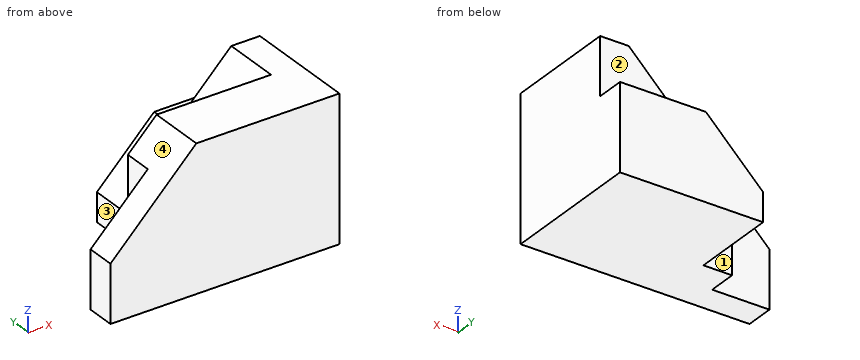
from build123d import *

# Parameters (mm, degrees)
SKETCH1_W           = 80
SKETCH1_H           = 50
BOSS_EXTRUDE1_DEPTH = 10
CUT_EXTRUDE1_DEPTH  = 10
BOSS_EXTRUDE2_DEPTH = 10
BOSS_EXTRUDE3_DEPTH = 20
BOSS_EXTRUDE4_DEPTH = 10


with BuildPart() as part:
    # Sketch1 → Boss-Extrude1 (new body)
    with BuildSketch(Plane(origin=(0, 0, 0), x_dir=(1, 0, 0), z_dir=(0, 1, 0))):
        with Locations((40, 25)):
            Rectangle(SKETCH1_W, SKETCH1_H)
    extrude(amount=BOSS_EXTRUDE1_DEPTH)

    # Sketch2 → Cut-Extrude1 (cut)
    with BuildSketch(Plane(origin=(0, 10, 0), x_dir=(1, 0, 0), z_dir=(0, 1, 0))):
        Polygon((0, 30), (30, 0), (0, 0), align=None)
    extrude(amount=-CUT_EXTRUDE1_DEPTH, mode=Mode.SUBTRACT)

    # Sketch3 → Boss-Extrude2 (add)
    with BuildSketch(Plane(origin=(0, 10, 0), x_dir=(1, 0, 0), z_dir=(0, 1, 0))):
        Polygon((80, 50), (80, 0), (30, 0), (20, 10), (20, 50), align=None)
    extrude(amount=BOSS_EXTRUDE2_DEPTH)

    # Sketch4 → Boss-Extrude3 (add)
    with BuildSketch(Plane(origin=(0, 20, 0), x_dir=(1, 0, 0), z_dir=(0, 1, 0))):
        Polygon((80, 50), (80, 0), (70, 0), (30, 40), (30, 50), align=None)
    extrude(amount=BOSS_EXTRUDE3_DEPTH)

    # Sketch5 → Boss-Extrude4 (add)
    with BuildSketch(Plane(origin=(0, 40, 0), x_dir=(1, 0, 0), z_dir=(0, 1, 0))):
        Polygon((80, 50), (80, 20), (50, 20), (30, 40), (30, 50), align=None)
    extrude(amount=BOSS_EXTRUDE4_DEPTH)


solid = part.part
Geometry check sheet. Reference: the model listing, model coordinates, mm. Face numbers are marked on the shaded views. A direction names the side the tool comes from. Coordinates: 2 decimals unless noted, no trailing zeros. Write each loop counter-clockwise with the first axis right and the second up, starting at its lowest first coordinate (ties: lowest second). Pieces come first, ordered by that corner, then holes. Notation, with made-up numbers: (-15.75, 12) -> (-4.75, 12) arc R23 cw to (-4.75, 33) -> close; hole circle Ø1 at (-8.5, -9). An arc over 180 degrees is marked (long way). One line per question, with ' | ' between items.
1. Cross-section at C-C on x = 43. Record the cut outline in (y, z).
Answers:
outline: (0, -50) -> (50, -50) -> (50, -27) -> (20, -27) -> (20, 0) -> (0, 0) -> close
2. Depth check by flat-ended pin: pin 1 Ø3 at (x, y) = (64, 45) entering from +Z; pin 2 Ø5 at (y, z) = (41.5, -44) entering from -X; pin 3 Ø12 at (x, z) = (25.5, -25.5) entering from +Y; pin 4 Ø1.5 at (x, y) = (29, 26.5) entering from -Z. Enter the tip coordinate at first touch or a pass-through.
Answers:
pin 1: stops at z = -20 | pin 2: stops at x = 30 | pin 3: stops at y = 20 | pin 4: passes through
3. Cross-section at B-B on y = 41. Record the cut outline in (x, z).
Answers:
outline: (30, -50) -> (80, -50) -> (80, -20) -> (50, -20) -> (30, -40) -> close
4. Cross-section at A-A on z = -41. Record the cut outline in (x, y), and give its area (3 significant figures).
Answers:
outline: (0, 0) -> (80, 0) -> (80, 50) -> (30, 50) -> (30, 20) -> (20, 20) -> (20, 10) -> (0, 10) -> close | area: 2,900 mm²
5. Set-up check for the marked faces 1, 2, 3 and 4: record each of +Z, -Z, +X, -X, +Y, -Y from which the full face is reachable in a straight line by a thin tool's end or side.
Answers:
face 1: +Z, -X, +Y | face 2: +Z, +X, -X, +Y | face 3: +Z, -Z, -X, +Y | face 4: +Z, -X, +Y, -Y
6. Thickness scan on probe 1 along Y at (x, z) = (35.5, -18.5); probe 2 along X at (y, z) = (14, -38); probe 3 along Y at (x, z) = (8.5, -38). Record the ranges inside material, lowest first. Write a range as from..to.
Answers:
probe 1: y = 0..20 | probe 2: x = 20..80 | probe 3: y = 0..10
7. Cross-section at D-D on z = -33. Record the cut outline in (x, y).
Answers:
outline: (0, 0) -> (80, 0) -> (80, 50) -> (37, 50) -> (37, 20) -> (20, 20) -> (20, 10) -> (0, 10) -> close
